For this review, take the finished solid that the model builds, in its own axes (mm). A direction names the side the tool comes from. Give positions to 0.01 mm unless a question says otherwise; leave off trailing zeros. Loops run counter-clockwise (first coordinate to the right, second up) from the corner with the lowest first, then second, coordinate; pieces in that order, holes last. Notation, with made-up numbers: (-12, 83) - (43, 83) arc R11 cw to (43, 87) - close; hole circle Ø9 at (15.25, -14.5). An arc over 180 degrees is marked (long way). Answer as CSV lines item,"result".
Autodesk Inventor part; units mm, degrees
ref_plane "YZ Plane" through (0, 0, 0) normal (1, 0, 0) x (0, 1, 0)
ref_plane "XZ Plane" through (0, 0, 0) normal (0, 1, 0) x (-1, 0, 0)
ref_plane "XY Plane" through (0, 0, 0) normal (0, 0, 1) x (1, 0, 0)
sketch "Skizze1" plane through (0, 0, 0) normal (0, 0, 1) x (1, 0, 0)
  line L0 (0, 0) -> (0, -50)
  line L1 (0, 0) -> (50, 0) construction
  line L2 (0, -50) -> (3, -50)
  line L3 (3, -50) -> (3, -3)
  line L4 (3, -3) -> (88, -3)
  line L5 (88, -3) -> (88, 0)
  line L6 (88, 0) -> (0, 0)
  dimension "d0" = 50
  dimension "d1" = 90
  dimension "d2" = 3
  dimension "d3" = 47
  dimension "d4" = 85
  dimension "d5" = 90
extrude "Extrusion1" add sketch "Skizze1" along normal mid plane 104
fillet "Rundung1" radius 52 2 edges at (88, -1.5, -52) (88, -1.5, 52)
sketch "Skizze2" plane through (3, -50, 52) normal (1, 0, 0) x (0, 0, -1)
  line L0 (3.5, 40) -> (8.5, 40)
  line L1 (8.5, 40) -> (8.5, 10)
  line L2 (8.5, 10) -> (3.5, 10)
  line L3 (3.5, 10) -> (3.5, 40)
  arc A0 (8.5, 40) -> (3.5, 40) centre (6, 40) ccw
  arc A1 (3.5, 10) -> (8.5, 10) centre (6, 10) ccw
  line L4 (0, 0) -> (0, 47)
  point P0 (52, 50)
  dimension "d9" = 5
  dimension "d10" = 30
  dimension "d27" = 6
extrude "Extrusion2" cut sketch "Skizze2" against normal blind 3
sketch "Skizze3" plane through (3, -50, 52) normal (1, 0, 0) x (0, 0, -1)
  line L0 (100.5, 40) -> (95.5, 40)
  line L1 (95.5, 40) -> (95.5, 10)
  line L2 (95.5, 10) -> (100.5, 10)
  line L3 (100.5, 10) -> (100.5, 40)
  arc A0 (100.5, 40) -> (95.5, 40) centre (98, 40) ccw
  arc A1 (95.5, 10) -> (100.5, 10) centre (98, 10) ccw
  line L4 (104, 47) -> (104, 0)
  point P0 (52, 50)
  dimension "d13" = 5
  dimension "d14" = 30
  dimension "d28" = 6
extrude "Extrusion3" cut sketch "Skizze3" against normal blind 3
sketch "Skizze4" plane through (0, 0, 52) normal (0, 1, 0) x (1, 0, 0)
  arc A0 (36, -0.5) -> (36, 104.5) centre (36, 52) ccw
  line L0 (36, 52) -> (36, -0.5) construction
  line L1 (36, 52) -> (88.5, 52) construction
  line L2 (36, 52) -> (36, 104.5) construction
  arc A1 (36, 4.5) -> (36, 99.5) centre (36, 52) ccw
  line L3 (36, 52) -> (36, 4.5) construction
  line L4 (36, 52) -> (83.5, 52) construction
  line L5 (36, 99.5) -> (0, 99.5)
  line L6 (0, 95.5) -> (0, 100.5)
  line L7 (36, 104) -> (3, 104)
  line L8 (36, -0.5) -> (0, -0.5)
  line L9 (0, -0.5) -> (0, 4.5)
  line L10 (36, 4.5) -> (0, 4.5)
  line L11 (0, 99.5) -> (0, 104.5)
  line L12 (0, 104.5) -> (36, 104.5)
  line L13 (0, 0) -> (0, 104)
  point P0 (0, 52)
  dimension "d17" = 52.5
  dimension "d18" = 90
  dimension "d19" = 180
  dimension "d20" = 47.5
  dimension "d21" = 90
extrude "Extrusion4" add sketch "Skizze4" along normal blind 1 and the other way blind 4 contours L8 L9 L10 A1 L5 L6 L11 L12 A0
properties part number "Glas und Flaschenboden"
1) Machinability: for faces 1 (the flat face through (1, -27, -52)), 2 (the flat face through (2, -25, 43.5)), 3 (the flat face through (42, 0, -1)), 4 (the flat face through (1, -27, 52)), which of the approach directions +Z, -Z, +X, -X, +Y, -Y give a long, thin tool a straight path to every point of the face, cutting with its end or side? Answer none if there is none.
From the geometry:
face 1,"-Z, +X, -X, -Y"
face 2,"+X, -X"
face 3,"-X, +Y"
face 4,"+Z, +X, -X, -Y"
2) Consider section B-B on z = 46. Write out the cut boundary in (x, y).
From the geometry:
outline,"(0, -50) - (3, -50) - (3, -42.5) - (0, -42.5) - close; (0, -7.5) - (3, -7.5) - (3, -3) - (47.84, -3) - (47.84, -4) - (61.3, -4) - (61.3, 1) - (47.84, 1) - (47.84, 0) - (0, 0) - close"
3) Draft analysis for pull direction X (two halves, no side actions). For faces 5 (the cylindrical face through (88.487, -1.535, -1.154)), 6 (the flat face through (43, -3, -1)), 7 (the cylindrical face through (83.49, 0.49, -1.04)), 8 (the cylindrical face through (1.5, -42.5, 46.1)), state which applies: pulls with the +X half, pulls with the -X half, needs draft (parallel to the pull), parting line crosses it, or undercut.
From the geometry:
face 5,"pulls with the +X half"
face 6,"undercut"
face 7,"pulls with the -X half"
face 8,"needs draft"
4) Consider section C-C on z = 0. Write out the cut boundary in (x, y).
From the geometry:
outline,"(0, -50) - (3, -50) - (3, -3) - (83.5, -3) - (83.5, -4) - (88.5, -4) - (88.5, 1) - (83.5, 1) - (83.5, 0) - (0, 0) - close"
5) Consider section D-D on x = 14.5. Write out the cut boundary in (y, z), and give its area (3 significant figures).
From the geometry:
outline,"(-4, -52.5) - (1, -52.5) - (1, -47.5) - (0, -47.5) - (0, 47.5) - (1, 47.5) - (1, 52.5) - (-4, 52.5) - (-4, 47.5) - (-3, 47.5) - (-3, -47.5) - (-4, -47.5) - close"
area,"335 mm^2"
6) Wall thickness on line 1 (X direction, y = -42, z = 42.5); line 2 (Y direction, x = 7.5, z = 43); line 3 (Z direction, x = 55, y = -1): over which ranges is each line inside the solid? List them lowest first. Write a range as from..to.
From the geometry:
line 1,"x = 0..3"
line 2,"y = -3..0"
line 3,"z = -48.94..48.94"
7) Insertion check: P1, Ø5, axis at x = 58.5, z = 31, coming from the -Y side; P2, Ø14, axis at y = -36.5, z = 13, coming from the +X side; P3, Ø3.5, axis at x = 1, y = -32, coming from the -Z side; P4, Ø1, axis at y = -19, z = -36, coming from the -X side. Each pin has a flat end and moves straight along its axis. Give the tip position at first contact, or say it passes through.
From the geometry:
P1,"stops at y = -3"
P2,"stops at x = 3"
P3,"stops at z = -52"
P4,"stops at x = 0"
8) Consider section A-A on y = -23.5. Write out the cut boundary in (x, z), and give its area (3 significant figures).
From the geometry:
outline,"(0, -52) - (3, -52) - (3, -48.5) - (0, -48.5) - close; (0, -43.5) - (3, -43.5) - (3, 43.5) - (0, 43.5) - close; (0, 48.5) - (3, 48.5) - (3, 52) - (0, 52) - close"
area,"282 mm^2"
